Source: CAD feature listing. Evaluate the final solid. Frame: model axes, mm. A direction names the side the tool comes from. Give positions to 0.01 mm unless a question says otherwise; leave off trailing zeros. Order: outer loops, then holes, each group sorted by start corner. A loop starts at its lowest first (then second) coordinate and runs counter-clockwise, first axis right, second up. Notation, with made-up numbers: (64, 86.25) -> (94, 86.25) arc R15 ccw to (94, 112.25) -> close; hole circle Ø11 at (89, 23.25). An arc over 180 degrees is marked (long way). Answer in a Markdown table with one row per item.
```python
from build123d import *

# Parameters (mm, degrees)
ESQUISSE1_R             = 11.1
ESQUISSE1_R_2           = 1.5
BOSS_EXTRU_1_DEPTH      = 2.35
ESQUISSE2_R             = 4.4
ESQUISSE2_R_2           = 3
BOSS_EXTRU_2_DEPTH      = 4
ESQUISSE3_R             = 1.43
ENL_V_MAT_EXTRU_1_DEPTH = 4
CHANFREIN2_SIZE         = 0.2
ESQUISSE4_R             = 1.5
ENL_V_MAT_EXTRU_2_DEPTH = 4
BOSS_EXTRU_3_START      = -2.35
ESQUISSE5_R             = 1.5
ESQUISSE5_R_2           = 0.75
BOSS_EXTRU_3_DEPTH      = 2.35


with BuildPart() as part:
    # Esquisse1 → Boss.-Extru.1 (new body)
    with BuildSketch(Plane.XY):
        Circle(ESQUISSE1_R)
        with Locations((0, 6.75)):
            Circle(ESQUISSE1_R_2, mode=Mode.SUBTRACT)
        with Locations((0, -6.75)):
            Circle(ESQUISSE1_R_2, mode=Mode.SUBTRACT)
    extrude(amount=BOSS_EXTRU_1_DEPTH)

    # Esquisse2 → Boss.-Extru.2 (add)
    with BuildSketch(Plane.XY.offset(2.35)):
        Circle(ESQUISSE2_R)
        Circle(ESQUISSE2_R_2, mode=Mode.SUBTRACT)
    extrude(amount=BOSS_EXTRU_2_DEPTH)

    # Esquisse3 → Enlèv. mat.-Extru.1 (cut)
    with BuildSketch(Plane.XY.offset(2.35)):
        Circle(ESQUISSE3_R)
    extrude(amount=-ENL_V_MAT_EXTRU_1_DEPTH, mode=Mode.SUBTRACT)

    # Chanfrein2
    chanfrein2_edges = [part.edges().sort_by_distance(p)[0] for p in [
        (-4.4, 0, 6.35),
    ]]
    chamfer(chanfrein2_edges, length=CHANFREIN2_SIZE)

    # Esquisse4 → Enlèv. mat.-Extru.2 (cut)
    with BuildSketch(Plane(origin=(0, 0, 0), x_dir=(-1, 0, 0), z_dir=(0, 0, -1))):
        with Locations((-6.75, 0)):
            Circle(ESQUISSE4_R)
        with Locations((6.75, 0)):
            Circle(ESQUISSE4_R)
    extrude(amount=-ENL_V_MAT_EXTRU_2_DEPTH, mode=Mode.SUBTRACT)

    # Esquisse5 → Boss.-Extru.3 (add)
    # profile 1 of 4: a face of its own
    with BuildSketch(Plane.XY.offset(2.35).offset(BOSS_EXTRU_3_START)):
        with Locations((-6.75, 0)):
            Circle(ESQUISSE5_R)
        with Locations((-6.75, 0)):
            Circle(ESQUISSE5_R_2, mode=Mode.SUBTRACT)
    # profile 2 of 4: a face of its own
    with BuildSketch(Plane.XY.offset(2.35).offset(BOSS_EXTRU_3_START)):
        with Locations((0, -6.75)):
            Circle(ESQUISSE5_R)
        with Locations((0, -6.75)):
            Circle(ESQUISSE5_R_2, mode=Mode.SUBTRACT)
    # profile 3 of 4: a face of its own
    with BuildSketch(Plane.XY.offset(2.35).offset(BOSS_EXTRU_3_START)):
        with Locations((6.75, 0)):
            Circle(ESQUISSE5_R)
        with Locations((6.75, 0)):
            Circle(ESQUISSE5_R_2, mode=Mode.SUBTRACT)
    # profile 4 of 4: a face of its own
    with BuildSketch(Plane.XY.offset(2.35).offset(BOSS_EXTRU_3_START)):
        with Locations((0, 6.75)):
            Circle(ESQUISSE5_R)
        with Locations((0, 6.75)):
            Circle(ESQUISSE5_R_2, mode=Mode.SUBTRACT)
    extrude(amount=BOSS_EXTRU_3_DEPTH)


solid = part.part
```
(1) Section query B-B (y = -6.75). Return the cut outline in (x, z), plus the area to 3 significant figures.
A:
| item | result |
|---|---|
| outline | (-8.81, 0) -> (-0.75, 0) -> (-0.75, 2.35) -> (-8.81, 2.35) -> close; (0.75, 0) -> (8.81, 0) -> (8.81, 2.35) -> (0.75, 2.35) -> close |
| area | 37.9 mm^2 |
(2) Pull-direction query (Y, two-part tool) for faces 3 (the cylindrical face through (-0.163, -7.482, 1.159)), 4 (the flat face through (5, 0, 2.35)), 5 (the cylindrical face through (5.97, 9.36, 1.16)); classes: +Y half, -Y half, draft (parallel to the pull), parting line (faces both ways), or undercut.
A:
| item | result |
|---|---|
| face 3 | undercut |
| face 4 | draft |
| face 5 | parting line |
(3) Access query for faces 1 (the cylindrical face through (-3, 0, 4)), 2 (the cylindrical face through (6, 0, 1)). Directions: +Z, -Z, +X, -X, +Y, -Y. A direction counts if a zero-diameter tool reaches every point of the face in a straight line with its end or side. Return the directions, or none.
A:
| item | result |
|---|---|
| face 1 | +Z |
| face 2 | +Z, -Z |
(4) First-contact query: pin 1 Ø2 at (y, z) = (8, 1) entering from -X; pin 2 Ø1.7 at (x, y) = (-6.75, 0) entering from +Z. Flat tips, straight axial feed; report the tip coordinate or a pass-through.
A:
| item | result |
|---|---|
| pin 1 | stops at x = -8.61 |
| pin 2 | stops at z = 2.35 |
(5) Ray query, probe 1 along Y at (x, z) = (0, 1.55); probe 2 along Z at (x, y) = (4, -6.5); probe 3 along Y at (x, z) = (-6.75, 1.6). Return the intervals inside material, ascending.
A:
| item | result |
|---|---|
| probe 1 | y = -11.1 to -7.5, -6 to -1.43, 1.43 to 6, 7.5 to 11.1 |
| probe 2 | z = 0 to 2.35 |
| probe 3 | y = -8.81 to -0.75, 0.75 to 8.81 |
(6) Section query A-A (x = 0). Return the cut outline in (y, z).
A:
| item | result |
|---|---|
| outline | (-11.1, 0) -> (-7.5, 0) -> (-7.5, 2.35) -> (-11.1, 2.35) -> close; (-6, 0) -> (-1.43, 0) -> (-1.43, 2.35) -> (-3, 2.35) -> (-3, 6.35) -> (-4.2, 6.35) -> (-4.4, 6.15) -> (-4.4, 2.35) -> (-6, 2.35) -> close; (1.43, 0) -> (6, 0) -> (6, 2.35) -> (4.4, 2.35) -> (4.4, 6.15) -> (4.2, 6.35) -> (3, 6.35) -> (3, 2.35) -> (1.43, 2.35) -> close; (7.5, 0) -> (11.1, 0) -> (11.1, 2.35) -> (7.5, 2.35) -> close |
(7) Section query C-C (z = 1). Return the cut outline in (x, y), plus the area to 3 significant figures.
A:
| item | result |
|---|---|
| outline | circle Ø22.2 at (0, 0); hole circle Ø1.5 at (-6.75, 0); hole circle Ø2.86 at (0, 0); hole circle Ø1.5 at (0, -6.75); hole circle Ø1.5 at (0, 6.75); hole circle Ø1.5 at (6.75, 0) |
| area | 374 mm^2 |
